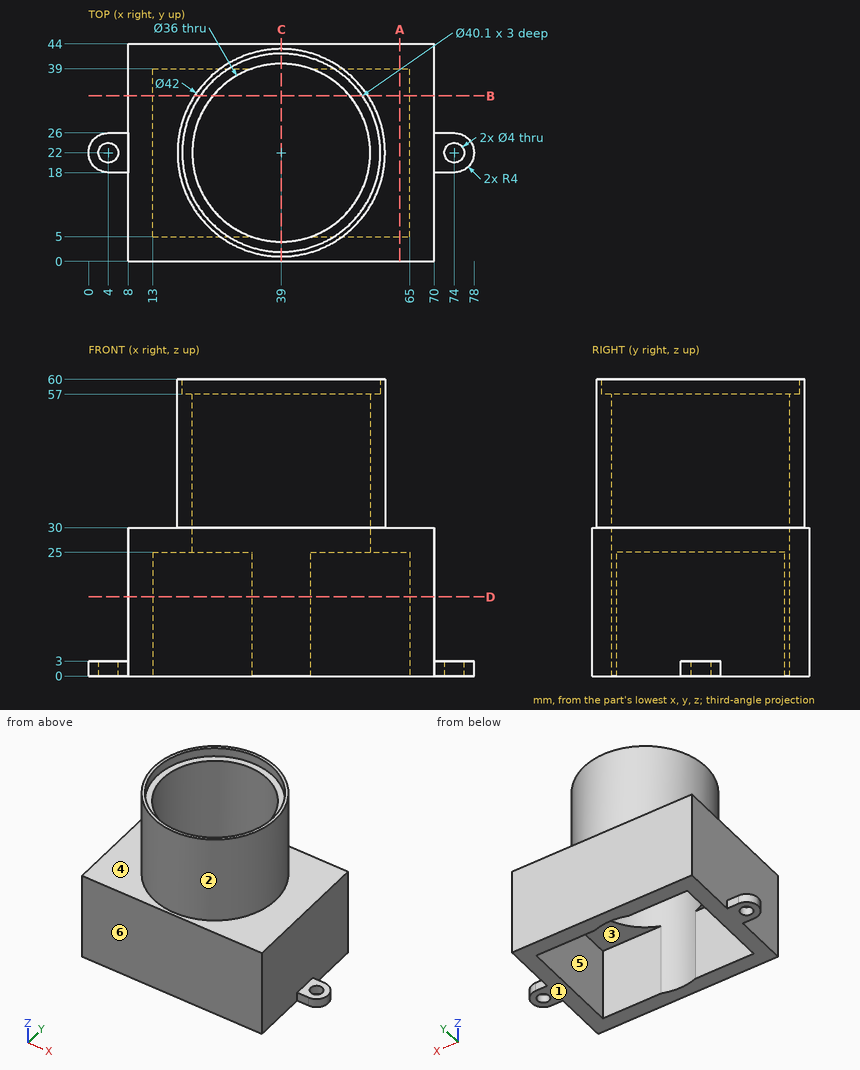
Geometry: see drawing. Coordinates: mm, zero at the bounding-box minimum. A direction names the side the tool comes from. Round coordinates to 2 decimals unless told otherwise and drop trailing zeros. Loops run counter-clockwise (first coordinate to the right, second up) from the corner with the lowest first, then second, coordinate; pieces in that order, holes last. Notation, with made-up numbers: (-11, 66.5) - (34, 66.5) arc R22 cw to (34, 103.5) - close; hole circle Ø1 at (16, 69). An arc over 180 degrees is marked (long way). Write item = value, one per line. Start each with the question number.
(1) Pin query (flat end, axial travel): pin 1 (3 mm diameter, centred on x = 58.5, y = 38.5, fed in from -Z); pin 2 (1 mm diameter, centred on y = 18, z = 40.5, fed in from -X); pin 3 (0.9 mm diameter, centred on x = 72.5, z = 1.5, fed in from +Y); pin 4 (10 mm diameter, centred on x = 59, y = 30, fed in from -Z). Return the tip coordinate at first contact, or that it passes through.
(2) Section query A-A, the plane x = 63. Output: boundary loops of the cut face in (y, z).
(3) Section query D-D, the plane z = 16. Output: boundary loops of the cut face in (x, y).
(4) Ray query, line 1 along X through (y, z) = (22, 2); line 2 along X through (y, z) = (17, 9); line 3 along Y through (x, z) = (74, 2.1). Return the intervals inside material, ascending. Write a range as from..to.
(5) Pull-direction query (X, two-part tool) for the marked faces 1, 2 and 3; classes: +X half, -X half, draft (parallel to the pull), parting line (faces both ways), or undercut.
(6) Set-up query: the marked faces 4, 5 and 6. Return all of +Z, -Z, +X, -X, +Y, -Y with unobstructed straight access to the full face (end or side cutting, diameter ignored); none if empty.
(7) Section query C-C, the plane x = 39. Output: boundary loops of the cut face in (y, z).
(8) Section query B-B, the plane y = 33.5. Output: boundary loops of the cut face in (x, z), plus the area to 4 significant figures.
Conclusion:
q1.pin_1 = 0
q1.pin_2 = 18.29
q1.pin_3 = 26
q1.pin_4 = 25
q2.outline = (0, 0) - (5, 0) - (5, 25) - (39, 25) - (39, 0) - (44, 0) - (44, 30) - (0, 30) - close
q3.outline = (8, 0) - (70, 0) - (70, 44) - (8, 44) - close; hole (13, 5) - (33.08, 5) arc R18 ccw to (44.92, 5) - (65, 5) - (65, 39) - (44.92, 39) arc R18 ccw to (33.08, 39) - (13, 39) - close
q4.line_1 = 0..2, 6..13, 65..72, 76..78
q4.line_2 = 8..13, 65..70
q4.line_3 = 18..20, 24..26
q5.face_1 = draft
q5.face_2 = parting line
q5.face_3 = undercut
q6.face_4 = +Z
q6.face_5 = -Z
q6.face_6 = +Z, -Z, +X, -X, -Y
q7.outline = (0, 0) - (4, 0) - (4, 57) - (1.95, 57) - (1.95, 60) - (1, 60) - (1, 30) - (0, 30) - close; (40, 0) - (44, 0) - (44, 30) - (43, 30) - (43, 60) - (42.05, 60) - (42.05, 57) - (40, 57) - close
q8.outline = (8, 0) - (13, 0) - (13, 25) - (25.15, 25) - (25.15, 57) - (22.58, 57) - (22.58, 60) - (21.43, 60) - (21.43, 30) - (8, 30) - close; (52.85, 25) - (65, 25) - (65, 0) - (70, 0) - (70, 30) - (56.57, 30) - (56.57, 60) - (55.42, 60) - (55.42, 57) - (52.85, 57) - close
q8.area = 629.5 mm2
